For this review, use the dimensioned drawing (mm, ordinates from the lowest corner) and the shaded views. Coordinates: 2 decimals unless noted, no trailing zeros. Loops run counter-clockwise (first coordinate to the right, second up) from the corner with the lowest first, then second, coordinate; pieces in that order, holes last. Notation, with made-up numbers: (67.5, 68) - (125.5, 68) arc R18 cw to (125.5, 99) - close; hole circle Ø10 at (18, 44.5). An arc over 180 degrees is marked (long way). Answer in a Markdown table with one row per item. Add a question column.
(1) The part is to be moulded in two halves that separate along X. For the marked faces 1 and 2, say which applies: released by +X, released by -X, zero draft, split by the parting line, or undercut.
(2) Clearance check with flat-ended pins moving along their axes: pin 1 (2 mm diameter, centred on x = 61.5, z = 71.5, fed in from +Y); pin 2 (1.5 mm diameter, centred on x = 32.5, z = 46, fed in from +Y); pin 3 (6 mm diameter, centred on x = 31, z = 53, fed in from +Y). State where each tip first meets the part, or that it passes through.
(3) We need section C-C, the plane z = 36.5. Write out the cut boundary in (x, y), plus the area to 3 significant figures.
(4) We need section A-A, the plane x = 35. Write out the cut boundary in (y, z).
(5) To check wall thickness, follow L1, parallel to X at y = 61, z = 67; L2, parallel to Y at x = 36, z = 16; L3, parallel to Y at x = 24.5, z = 73. State the ranges of each line that lie inside material, in increasing order. Write a range as [from, to].
(6) We need section D-D, the plane z = 60. Write out the cut boundary in (x, y), plus the area to 3 significant figures.
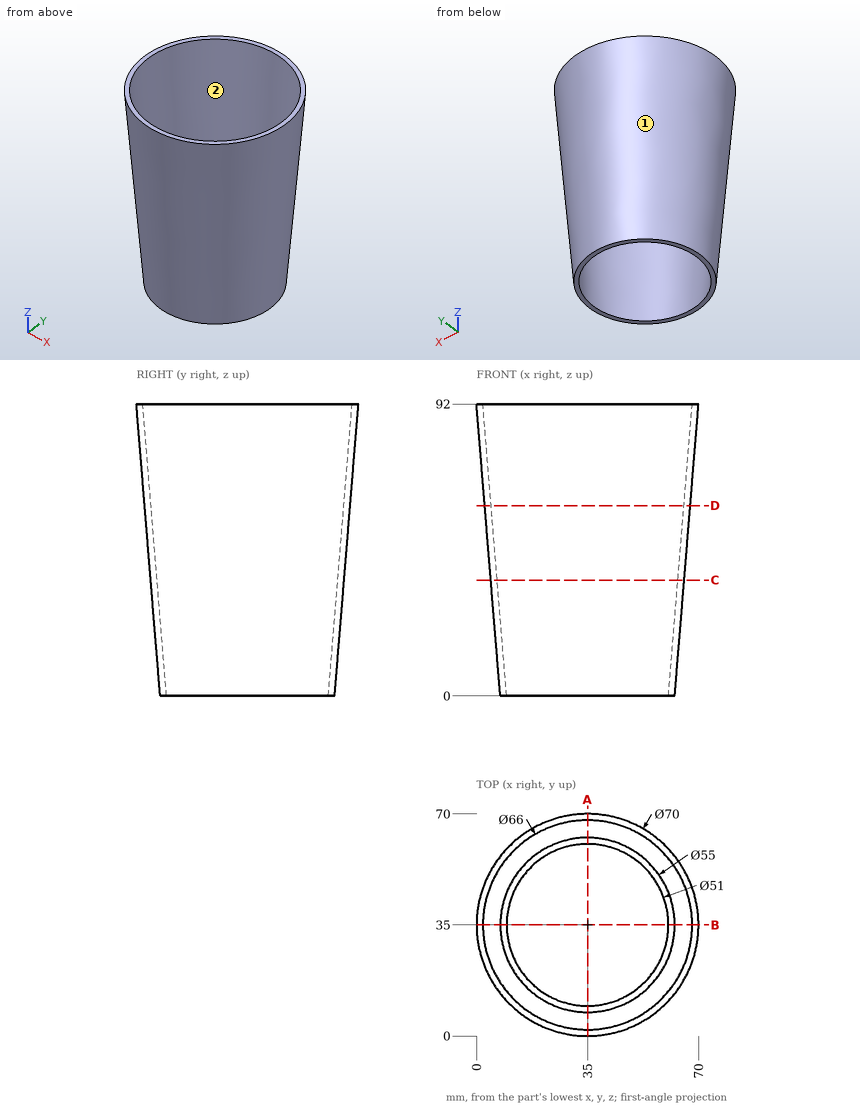
Responses:
| question | item | result |
|---|---|---|
| 1 | face 1 | split by the parting line |
| 1 | face 2 | undercut |
| 2 | pin 1 | stops at y = 56.47 |
| 2 | pin 2 | stops at y = 66.23 |
| 2 | pin 3 | stops at y = 66.94 |
| 3 | outline | circle Ø60.95 at (35, 35); hole circle Ø56.95 at (35, 35) |
| 3 | area | 370 mm2 |
| 4 | outline | (0, 92) - (7.5, 0) - (9.5, 0) - (2, 92) - close; (60.5, 0) - (62.5, 0) - (70, 92) - (68, 92) - close |
| 5 | L1 | x = [14.74, 18.19], [51.81, 55.26] |
| 5 | L2 | y = [6.21, 8.21], [61.79, 63.79] |
| 5 | L3 | y = [3.24, 5.35], [64.65, 66.76] |
| 6 | outline | circle Ø64.78 at (35, 35); hole circle Ø60.78 at (35, 35) |
| 6 | area | 394 mm2 |
